The model under review builds one solid part; all positions refer to its coordinate system, in mm. A direction names the side the tool comes from. Round coordinates to 2 decimals unless told otherwise and drop trailing zeros. Order: outer loops, then holes, each group sorted by start corner. A loop starts at its lowest first (then second) coordinate and runs counter-clockwise, first axis right, second up.
1) Consider section A-A (y = 1.5). Give the boundary of the cut face in (x, z), then the cut area to 3 significant figures.
2) Machinability: for faces 5 (the face through (0, -5, 15.24)), 6 (the face through (0, -10, 3.81)), 7 (the face through (0, -8.89, 3)), which of the approach directions +Z, -Z, +X, -X, +Y, -Y give a long, thin tool a straight path to every point of the face, cutting with its end or side? Answer none if there is none.
3) Clearance check with flat-ended pins moving along their axes: P1, Ø0.6, axis at x = 1, y = -9.5, coming from the +Z side; P2, Ø1.4, axis at y = -9.5, z = 3.5, coming from the -X side; P3, Ø1.4, axis at x = -1, z = 3, coming from the +Y side; P4, Ø6, axis at x = 12, z = 19.5, coming from the -Y side. State where each tip first meets the part, or that it passes through.
4) Consider section C-C (y = 4.25). Give the boundary of the cut face in (x, z), then the cut area to 3 significant figures.
5) Consider section D-D (x = 17). Give the boundary of the cut face in (y, z).
6) Mouldability with a two-part tool opening along Z and no side actions: class faces 1 (the face through (2, -2, 27.94)), 2 (the face through (-2.214, -7.291, 9.207)), 3 (the face through (-12, 4, 8)), 4 (the face through (-3.83, -2.937, 21.501)) as pulls with the +Z half, pulls with the -Z half, needs draft (parallel to the pull), parting line crosses it, or undercut.
7) To check wall thickness, follow L1, parallel to Y at x = 0, z = 18.75; L2, parallel to Y at x = 0, z = 6; L3, parallel to X at y = -8.25, z = 1.75. State the ranges of each line that lie inside material, in increasing order.
8) Consider section B-B (z = 9.25). Give the boundary of the cut face in (x, y) (3 decimals), then the cut area to 3 significant figures.
from build123d import *
from build123d import SkipClean  # not in build123d's __all__

# Parameters (mm, degrees)
F0_R      = 7.62
F1_DEPTH  = 15.24
F3_DEPTH  = 20.32
F5_COUNT  = 2
F6_W      = 5.0799995622
F6_H      = 2.54
F7_DEPTH  = 10.16
F8_W      = 5.0799995622
F8_H      = 1.27
F9_DEPTH  = 1.27
F10_R     = 2.54
F11_DEPTH = 15.241
F12_R     = 4.826
F12_R_2   = 2.54
F13_DEPTH = 12.7


with BuildPart() as f1:
    # F0 (on Top) → F1 (new body)
    with BuildSketch(Plane.XY):
        Circle(F0_R)
    extrude(amount=F1_DEPTH)



with BuildPart() as f3:
    # F2 (on Right) → F3 (new body)
    with BuildSketch(Plane.YZ):
        Polygon((-7.62, 15.24), (0, 0), (7.62, 0), align=None)
    extrude(amount=F3_DEPTH)


with BuildPart() as f1_1:
    add(f1.part, clean=False)

    with SkipClean():  # cleaning this boolean's faces spoils the solid; the shape is the same uncleaned
        add(f3.part)  # F5 merges F3
    # F5: F3 ×2 about axis
    f5_axis = Axis((0, 0, 17.5851359963), (0, 0, 1))
    with SkipClean():  # cleaning this boolean's faces spoils the solid; the shape is the same uncleaned
        for i in range(1, F5_COUNT):
            add(f3.part.rotate(f5_axis, i * 360 / F5_COUNT), clean=False)

    # F6 (on Front) → F7 (join)
    with BuildSketch(Plane.XZ):
        with Locations((0, 1.27)):
            Rectangle(F6_W, F6_H)
    with SkipClean():  # cleaning this boolean's faces spoils the solid; the shape is the same uncleaned
        extrude(amount=F7_DEPTH)

    # F8 (on face) → F9 (join)
    with BuildSketch(Plane.XY.offset(2.54)):
        with Locations((0, -9.525)):
            Rectangle(F8_W, F8_H)
    with SkipClean():  # cleaning this boolean's faces spoils the solid; the shape is the same uncleaned
        extrude(amount=F9_DEPTH)

    # F10 (on face) → F11 (cut, through all)
    with BuildSketch(Plane.XY.offset(15.24)):
        Circle(F10_R)
    with SkipClean():  # cleaning this boolean's faces spoils the solid; the shape is the same uncleaned
        extrude(amount=-F11_DEPTH, mode=Mode.SUBTRACT)

    # F12 (on face) → F13 (join)
    with BuildSketch(Plane.XY.offset(15.24)):
        Circle(F12_R)
        Circle(F12_R_2, mode=Mode.SUBTRACT)
    with SkipClean():  # cleaning this boolean's faces spoils the solid; the shape is the same uncleaned
        extrude(amount=F13_DEPTH)


solid = f1_1.part
Answer below:
1. outline: (-20.32, 3) - (-7.47, 3) - (-7.47, 0) - (-2.05, 0) - (-2.05, 27.94) - (-4.59, 27.94) - (-4.59, 15.24) - (-7.47, 15.24) - (-7.47, 9.12) - (-20.32, 9.12) - close; (2.05, 0) - (20.32, 0) - (20.32, 6.12) - (7.47, 6.12) - (7.47, 15.24) - (4.59, 15.24) - (4.59, 27.94) - (2.05, 27.94) - close
1. area: 387 mm2
2. face 5: +Z
2. face 6: +Z, +X, -X, -Y
2. face 7: +Z, +X, -X
3. P1: stops at z = 3.81
3. P2: stops at x = -2.54
3. P3: stops at y = 7.61
3. P4: passes through
4. outline: (-20.32, 8.5) - (-6.32, 8.5) - (-6.32, 0) - (20.32, 0) - (20.32, 3.37) - (6.32, 3.37) - (6.32, 15.24) - (2.29, 15.24) - (2.29, 27.94) - (-2.29, 27.94) - (-2.29, 15.24) - (-6.32, 15.24) - (-6.32, 11.87) - (-20.32, 11.87) - close
4. area: 345 mm2
5. outline: (-7.62, 15.24) - (0, 0) - (7.62, 0) - close
6. face 1: pulls with the +Z half
6. face 2: undercut
6. face 3: pulls with the -Z half
6. face 4: needs draft
7. L1: y = -4.83 to -2.54, 2.54 to 4.83
7. L2: y = -7.62 to -2.54, 2.54 to 7.62
7. L3: x = -2.54 to 2.54
8. outline: (-20.32, 1.63) - (-7.444, 1.63) arc R7.62 ccw to (6.056, -4.625) - (20.32, -4.625) - (20.32, -1.63) - (7.444, -1.63) arc R7.62 ccw to (-6.056, 4.625) - (-20.32, 4.625) - close; hole circle Ø5.08 at (0, 0)
8. area: 243 mm2
